```python
from build123d import *

# Parameters (mm, degrees)
AUFSATZ_LINEAR_AUSTRAGEN1_DEPTH      = 1.33
SKIZZE2_R                            = 3.4
SKIZZE2_R_2                          = 2.3
AUFSATZ_LINEAR_AUSTRAGEN2_DEPTH      = 2.3
AUFSATZ_LINEAR_AUSTRAGEN2_DEPTH_BACK = 1.33
SKIZZE3_R                            = 1.25
SCHNITT_LINEAR_AUSTRAGEN1_DEPTH      = 2.33
SKIZZE4_R                            = 2.35
SCHNITT_LINEAR_AUSTRAGEN2_DEPTH      = 1.1
SKIZZE5_R                            = 0.45
SCHNITT_LINEAR_AUSTRAGEN3_DEPTH      = 2.33


with BuildPart() as part:
    # Skizze1 → Aufsatz-Linear austragen1 (new body)
    with BuildSketch(Plane.XY):
        with BuildLine():
            Line((-16.79191458, 1.869621687), (-1.9, 3))
            Line((-1.9, 3), (-1.9, 6.5))
            ThreePointArc((-1.9, 6.5), (0, 8.4), (1.9, 6.5))
            Line((1.9, 6.5), (1.9, 3))
            Line((1.9, 3), (16.79191458, 1.869621687))
            ThreePointArc((16.79191458, 1.869621687), (18.525, 0), (16.79191458, -1.869621687))
            Line((16.79191458, -1.869621687), (1.9, -3))
            Line((1.9, -3), (1.9, -6.5))
            ThreePointArc((1.9, -6.5), (0, -8.4), (-1.9, -6.5))
            Line((-1.9, -6.5), (-1.9, -3))
            Line((-1.9, -3), (-16.79191458, -1.869621687))
            ThreePointArc((-16.79191458, -1.869621687), (-18.525, 0), (-16.79191458, 1.869621687))
        make_face()
    extrude(amount=AUFSATZ_LINEAR_AUSTRAGEN1_DEPTH)

    # Skizze2 → Aufsatz-Linear austragen2 (add, two sides)
    with BuildSketch(Plane.XY.offset(1.33)) as aufsatz_linear_austragen2_sk:
        Circle(SKIZZE2_R)
        Circle(SKIZZE2_R_2, mode=Mode.SUBTRACT)
    extrude(amount=AUFSATZ_LINEAR_AUSTRAGEN2_DEPTH)
    extrude(aufsatz_linear_austragen2_sk.sketch, amount=-AUFSATZ_LINEAR_AUSTRAGEN2_DEPTH_BACK)

    # Skizze3 → Schnitt-Linear austragen1 (cut, through all)
    with BuildSketch(Plane.XY.offset(1.33)):
        Circle(SKIZZE3_R)
    extrude(amount=-SCHNITT_LINEAR_AUSTRAGEN1_DEPTH, mode=Mode.SUBTRACT)

    # Skizze4 → Schnitt-Linear austragen2 (cut)
    with BuildSketch(Plane(origin=(0, 0, 0), x_dir=(-1, 0, 0), z_dir=(0, 0, -1))):
        Circle(SKIZZE4_R)
    extrude(amount=-SCHNITT_LINEAR_AUSTRAGEN2_DEPTH, mode=Mode.SUBTRACT)

    # Skizze5 → Schnitt-Linear austragen3 (cut, through all)
    with BuildSketch(Plane.XY.offset(1.33)):
        with Locations((0, 6.5)):
            Circle(SKIZZE5_R)
        with Locations((-16.65, 0)):
            Circle(SKIZZE5_R)
        with Locations((0, 4.5)):
            Circle(SKIZZE5_R)
        with Locations((-14.65, 0)):
            Circle(SKIZZE5_R)
        with Locations((-12.65, 0)):
            Circle(SKIZZE5_R)
        with Locations((-10.65, 0)):
            Circle(SKIZZE5_R)
        with Locations((-8.65, 0)):
            Circle(SKIZZE5_R)
        with Locations((-6.65, 0)):
            Circle(SKIZZE5_R)
        with Locations((-4.65, 0)):
            Circle(SKIZZE5_R)
        with Locations((0, -4.5)):
            Circle(SKIZZE5_R)
        with Locations((0, -6.5)):
            Circle(SKIZZE5_R)
        with Locations((4.65, 0)):
            Circle(SKIZZE5_R)
        with Locations((6.65, 0)):
            Circle(SKIZZE5_R)
        with Locations((8.65, 0)):
            Circle(SKIZZE5_R)
        with Locations((10.65, 0)):
            Circle(SKIZZE5_R)
        with Locations((12.65, 0)):
            Circle(SKIZZE5_R)
        with Locations((14.65, 0)):
            Circle(SKIZZE5_R)
        with Locations((16.65, 0)):
            Circle(SKIZZE5_R)
    extrude(amount=-SCHNITT_LINEAR_AUSTRAGEN3_DEPTH, mode=Mode.SUBTRACT)


solid = part.part
```
CAD build for the part. Positions are in the model's coordinates, mm. A direction names the side the tool comes from. Round coordinates to 2 decimals unless told otherwise and drop trailing zeros. Order: outer loops, then holes, each group sorted by start corner. A loop starts at its lowest first (then second) coordinate and runs counter-clockwise, first axis right, second up. Notation, with made-up numbers: (-4, 15) -> (26, 15) arc R15 ccw to (26, 39) -> close; hole circle Ø2 at (-40, 60). An arc over 180 degrees is marked (long way). Write item = value, one per line.
(1) Cut at D-D (z = 2.6). Write the cut outline in (x, y).
Answers follow:
outline = circle Ø6.8 at (0, 0); hole circle Ø4.6 at (0, 0)
(2) Pull direction Y, two halves, no side cores. Call faces 1 (the flat face through (3, 2, 1.33)), 2 (the cylindrical face through (-0.059, -4.054, 0.674)), 3 (the cylindrical face through (-0.74, -3.32, 2.46)): +Y half, -Y half, draft (parallel to the pull), parting line (faces both ways), or undercut.
Answers follow:
face_1 = draft
face_2 = undercut
face_3 = parting line
(3) 3-axis set-ups, long thin cutter, end or side, ignore diameter. For faces 4 (the flat face through (-1.9, -5, 1)), 5 (the cylindrical face through (0, 8.4, 0.7)), 6 (the flat face through (-1, -1, 1.1)), 7 (the flat face through (1.9, -5, 1)), 8 (the flat face through (-1, -1, 1.33)): which of +Z, -Z, +X, -X, +Y, -Y reach the whole face in a straight line?
Answers follow:
face_4 = +Z, -Z, -X, -Y
face_5 = +Z, -Z, +Y
face_6 = -Z
face_7 = +Z, -Z, +X, -Y
face_8 = +Z
(4) Flat gauge pins, fed straight in: P1, Ø1.1, axis at y = -4.5, z = 0.5, coming from the +X side; P2, Ø1.4, axis at x = -0.5, y = -1, coming from the +Z side; P3, Ø3, axis at x = -6, y = -5.5, coming from the +Z side; P4, Ø6, axis at x = 14, y = 2.5, coming from the -Z side. Where does each tip first touch, or does it go through?
Answers follow:
P1 = 1.9
P2 = 1.33
P3 = through
P4 = 0
(5) Cut at C-C (x = -10.65). Write the cut outline in (y, z).
Answers follow:
outline = (-2.34, 0) -> (-0.45, 0) -> (-0.45, 1.33) -> (-2.34, 1.33) -> close; (0.45, 0) -> (2.34, 0) -> (2.34, 1.33) -> (0.45, 1.33) -> close
(6) Cut at B-B (z = 0.6). State how many separate pieces and enclosed holes the cut face has, plus the area to 3 significant figures.
Answers follow:
separate_pieces = 1
enclosed_holes = 19
area = 187 mm²
(7) Drill centre lines: L1, parallel to Y at x = 0, z = 2.55; L2, parallel to Z at x = 0, y = -7.5; L3, parallel to Z at x = 1, y = 1.75. Where is each one in solid material? Low to high.
Answers follow:
L1 = -3.4 to -2.3, 2.3 to 3.4
L2 = 0 to 1.33
L3 = 1.1 to 1.33
(8) Cut at A-A (y = -4.5). Write the cut outline in (x, z), plus the area to 3 significant figures.
Answers follow:
outline = (-1.9, 0) -> (-0.45, 0) -> (-0.45, 1.33) -> (-1.9, 1.33) -> close; (0.45, 0) -> (1.9, 0) -> (1.9, 1.33) -> (0.45, 1.33) -> close
area = 3.86 mm²
